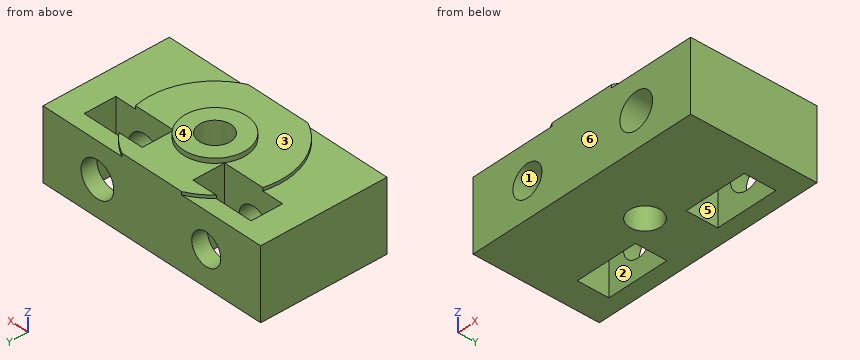
from build123d import *

# Parameters (mm, degrees)
SKETCH_1_W               = 30
SKETCH_1_H               = 16
SKETCH_1_R               = 2
EXTRUDE_1_DEPTH          = 8.9
SKETCH_2_R               = 2
SKETCH_2_R_2             = 2.25
CUT_EXTRUDE_1_DEPTH      = 18
SKETCH_3_W               = 8
SKETCH_3_H               = 4
CUT_EXTRUDE_2_DEPTH      = 2
CUT_EXTRUDE_2_DEPTH_BACK = 9.9
CUT_EXTRUDE_4_DEPTH      = 10.9


with BuildPart() as part:
    # Эскиз1 → Бобышка-Вытянуть1 (new body)
    with BuildSketch(Plane.XY):
        Rectangle(SKETCH_1_W, SKETCH_1_H)
        Circle(SKETCH_1_R, mode=Mode.SUBTRACT)
    extrude(amount=EXTRUDE_1_DEPTH)

    # Эскиз5 → Повернуть1 (revolve)
    with BuildSketch(Plane(origin=(0, 0, 0), x_dir=(-1, 0, 0), z_dir=(0, 1, 0))):
        Polygon((2, 8.9), (2, 9.9), (4, 9.9), (4, 9.3), (9, 9.3), (9, 8.9), align=None)
    revolve(axis=Axis((0, 0, 8.9), (0, 0, -1)))

    # Эскиз2 → Вырез-Вытянуть1 (cut, through all)
    with BuildSketch(Plane.XZ.offset(8)):
        with Locations((-7.5, 4.45)):
            Circle(SKETCH_2_R)
        with Locations((7.5, 4.45)):
            Circle(SKETCH_2_R_2)
    extrude(amount=-CUT_EXTRUDE_1_DEPTH, mode=Mode.SUBTRACT)

    # Эскиз3 → Вырез-Вытянуть2 (cut, two sides)
    with BuildSketch(Plane.XY.offset(8.9)) as cut_extrude_2_sk:
        with Locations((-7.5, 4)):
            Rectangle(SKETCH_3_W, SKETCH_3_H)
        with Locations((7.5, 4)):
            Rectangle(SKETCH_3_W, SKETCH_3_H)
    extrude(amount=CUT_EXTRUDE_2_DEPTH, mode=Mode.SUBTRACT)
    extrude(cut_extrude_2_sk.sketch, amount=-CUT_EXTRUDE_2_DEPTH_BACK, mode=Mode.SUBTRACT)

    # Эскиз7 → Вырез-Вытянуть4 (cut, through all)
    with BuildSketch(Plane(origin=(0, 0, 0), x_dir=(-1, 0, 0), z_dir=(0, 0, -1))):
        with BuildLine():
            Line((-4.123105626, 8), (4.123105626, 8))
            ThreePointArc((4.123105626, 8), (0, 9), (-4.123105626, 8))
        make_face()
        with BuildLine():
            ThreePointArc((-4.123105626, -8), (0, -9), (4.123105626, -8))
            Line((4.123105626, -8), (-4.123105626, -8))
        make_face()
    extrude(amount=-CUT_EXTRUDE_4_DEPTH, mode=Mode.SUBTRACT)


solid = part.part
Input: part model. Units: mm. Frame: model coordinates. Face numbers are marked on the shaded views. A direction names the side the tool comes from. Give positions to 0.01 mm unless a question says otherwise; leave off trailing zeros. Order: outer loops, then holes, each group sorted by start corner. A loop starts at its lowest first (then second) coordinate and runs counter-clockwise, first axis right, second up. Notation, with made-up numbers: (9, -36) - (24, -36) arc R4 cw to (24, -29) - close; hole circle Ø11 at (56.5, 62). An arc over 180 degrees is marked (long way). Answer as a JSON object with one key per item and string values. Group by question number.
Q1. Mould query, pull axis Y, two halves, no side actions, for the marked faces 4, 5 and 6. Classes: pulls with the +Y half, pulls with the -Y half, needs draft (parallel to the pull), parting line crosses it, or undercut.
Q2. First-contact query: pin 1 Ø2.5 at (x, z) = (-7.5, 4.45) entering from +Y; pin 2 Ø2 at (x, y) = (-4.5, -3.5) entering from -Z; pin 3 Ø8.5 at (x, y) = (9, -1) entering from +Z. Flat tips, straight axial feed; report the tip coordinate or a pass-through.
Q3. Cut plane D-D, the plane y = 0. Output: boundary loops of the cut face in (x, z).
Q4. Cut plane A-A, the plane x = 0. Output: boundary loops of the cut face in (y, z).
Q5. Cut plane C-C, the plane y = -6. Output: boundary loops of the cut face in (x, z), then the cut area to 3 significant figures.
Q6. Line query: probe 1 along X at (y, z) = (-3.5, 4.5); probe 2 along X at (y, z) = (3.25, 7.75); probe 3 along Y at (x, z) = (0, 4.5). Output: solid intervals per line, ascending.
Q7. Set-up query: the marked faces 1, 2 and 3. Return all of +Z, -Z, +X, -X, +Y, -Y with unobstructed straight access to the full face (end or side cutting, diameter ignored); none if empty.
Q8. Cut plane B-B, the plane z = 4.45. Count the separate pieces of the cut face and the enclosed holes in it, then the cut area to 3 significant figures.
Results:
{
 "1": {"face 4": "needs draft", "face 5": "undercut", "face 6": "pulls with the -Y half"},
 "2": {"pin 1": "through", "pin 2": "z = 0", "pin 3": "z = 9.3"},
 "3": {"outline": "(-15, 0) - (-2, 0) - (-2, 9.9) - (-4, 9.9) - (-4, 9.3) - (-9, 9.3) - (-9, 8.9) - (-15, 8.9) - close; (2, 0) - (15, 0) - (15, 8.9) - (9, 8.9) - (9, 9.3) - (4, 9.3) - (4, 9.9) - (2, 9.9) - close; hole circle Ø4 at (-7.5, 4.45); hole circle Ø4.5 at (7.5, 4.45)"},
 "4": {"outline": "(-8, 0) - (-2, 0) - (-2, 9.9) - (-4, 9.9) - (-4, 9.3) - (-8, 9.3) - close; (2, 0) - (8, 0) - (8, 9.3) - (4, 9.3) - (4, 9.9) - (2, 9.9) - close"},
 "5": {"outline": "(-15, 0) - (15, 0) - (15, 8.9) - (6.71, 8.9) - (6.71, 9.3) - (-6.71, 9.3) - (-6.71, 8.9) - (-15, 8.9) - close; hole circle Ø4 at (-7.5, 4.45); hole circle Ø4.5 at (7.5, 4.45)", "area": "244 mm^2"},
 "6": {"probe 1": "-15 to -9.5, -5.5 to 5.25, 9.75 to 15", "probe 2": "-15 to -11.5, -3.5 to 3.5, 11.5 to 15", "probe 3": "-8 to -2, 2 to 8"},
 "7": {"face 1": "+Y, -Y", "face 2": "+Z, -Z", "face 3": "+Z"},
 "8": {"separate pieces": "3", "enclosed holes": "1", "area": "301 mm^2"}
}
